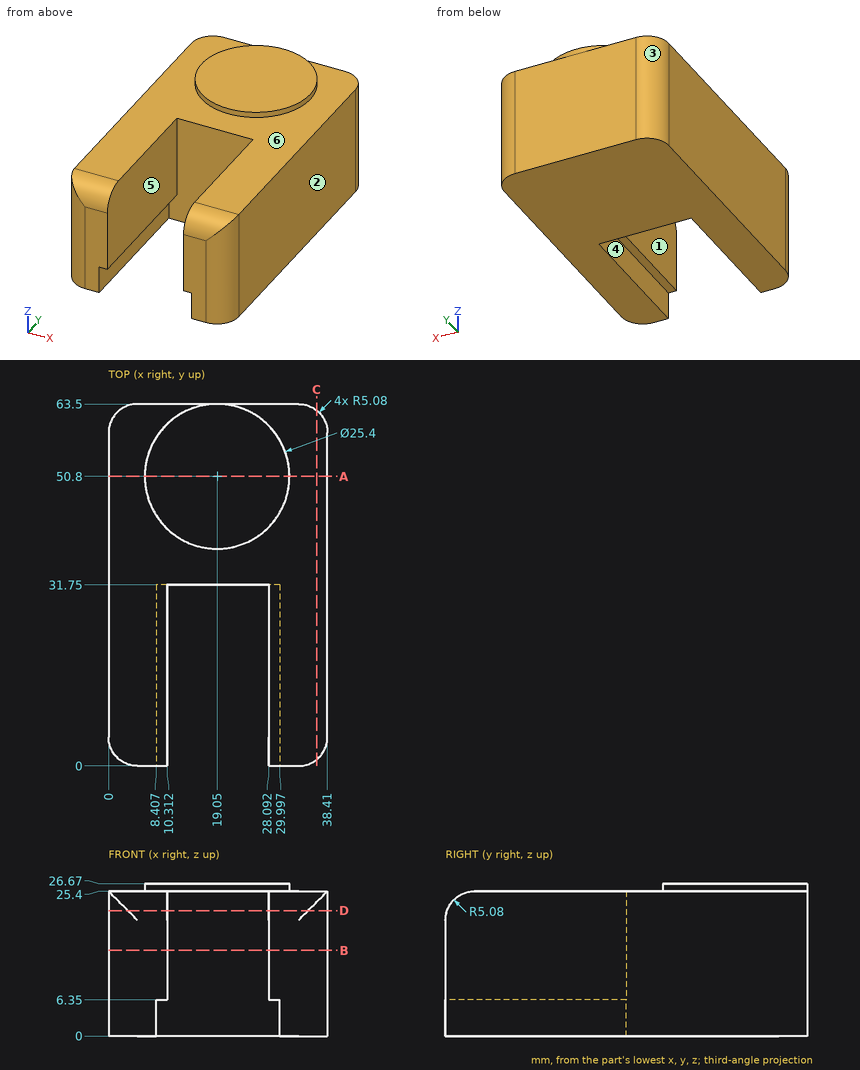
Verification items for this drawing (mm, ordinates from the low corner). A direction names the side the tool comes from. Give positions to 0.01 mm unless a question says otherwise; leave off trailing zeros. Loops run counter-clockwise (first coordinate to the right, second up) from the corner with the lowest first, then second, coordinate; pieces in that order, holes last. Notation, with made-up numbers: M 2.25,26 L 26.25,26 A31 ccw 26.25,51 Z; hole C 39,71.25 d10. An arc over 180 degrees is marked long. Return JSON: item names as keys, results as strings. Group by question number.
1. Tool access check on the marked faces 1 and 2. Record the directions out of +Z, -Z, +X, -X, +Y, -Y that give a thin tool (end or side, any length) a straight path to the whole face; none if there is none.
2. Thickness scan on L1, parallel to X at y = 28, z = 7.5; L2, parallel to X at y = 6, z = 4; L3, parallel to Z at x = 31.5, y = 55. Record the ranges inside material, lowest first.
3. Cross-section at C-C on x = 36.5. Record the boundary of the cut face in (y, z), plus the area to 3 significant figures.
4. Cross-section at A-A on y = 50.8. Record the boundary of the cut face in (x, z), plus the area to 3 significant figures.
5. Cross-section at B-B on z = 15. Record the boundary of the cut face in (x, y), plus the area to 3 significant figures.
6. Cross-section at D-D on z = 22. Record the boundary of the cut face in (x, y).
7. Go/stop test with a flat-tipped pin: pin 1 (1 mm diameter, centred on x = 29, y = 20.5, fed in from -Z). Record where the tip stops, or that it passes through.
8. Mould release check, pull along X, two halves, no side actions. Record for the marked faces 3, 4, 5 and 6: released by +X, released by -X, zero draft, split by the parting line, or undercut.
Return value:
{
 "1": {"face 1": "+Z, -Z, -Y", "face 2": "+Z, -Z, +X, +Y, -Y"},
 "2": {"L1": "0 to 10.31, 28.09 to 38.41", "L2": "0 to 8.41, 30 to 38.41", "L3": "0 to 25.4"},
 "3": {"outline": "M 1.11,0 L 62.39,0 L 62.39,25.4 L 5.08,25.4 A5.08 ccw 1.11,23.49 Z", "area": "1,550 mm^2"},
 "4": {"outline": "M 0,0 L 38.41,0 L 38.41,25.4 L 31.75,25.4 L 31.75,26.67 L 6.35,26.67 L 6.35,25.4 L 0,25.4 Z", "area": "1,010 mm^2"},
 "5": {"outline": "M 0,5.08 A5.08 ccw 5.08,0 L 10.31,0 L 10.31,31.75 L 28.09,31.75 L 28.09,0 L 33.33,0 A5.08 ccw 38.41,5.08 L 38.41,58.42 A5.08 ccw 33.33,63.5 L 5.08,63.5 A5.08 ccw 0,58.42 Z", "area": "1,850 mm^2"},
 "6": {"outline": "M 0,5.08 A5.08 ccw 3.4,0.29 L 10.31,0.29 L 10.31,31.75 L 28.09,31.75 L 28.09,0.29 L 35.01,0.29 A5.08 ccw 38.41,5.08 L 38.41,58.42 A5.08 ccw 33.33,63.5 L 5.08,63.5 A5.08 ccw 0,58.42 Z"},
 "7": {"pin 1": "z = 6.35"},
 "8": {"face 3": "released by -X", "face 4": "undercut", "face 5": "undercut", "face 6": "zero draft"}
}
